The listing builds one solid part. Answer for the finished solid, in the listing's coordinates (mm). A direction names the side the tool comes from. Round coordinates to 2 decimals unless told otherwise and drop trailing zeros. Write each loop counter-clockwise with the first axis right and the second up, starting at its lowest first coordinate (ties: lowest second). Pieces come first, ordered by that corner, then holes.
(1) A cutting plane is placed at C-C, the plane y = 32. Give the vertices of the cut face in (x, z).
(2) A cutting plane is placed at B-B, the plane x = 23. Give the vertices of the cut face in (y, z).
(3) A cutting plane is placed at D-D, the plane z = 0.6. Give the vertices of the cut face in (x, y).
(4) For faces 5 (the face through (19, 8, 2)), 6 (the face through (13, 18, 3)), determine the directions among +Z, -Z, +X, -X, +Y, -Y from which every point of the face is accessible in a straight line to the end or side of a thin tool.
(5) This flat-tipped pin is pushed along its axis until it touches: pin 1 Ø4 at (x, y) = (18.5, 6) entering from +Z. Where does it stop, or does it pass through?
(6) Find the intervals of material crossed by probe 1 along X at (y, z) = (33, 1.5); probe 2 along Y at (x, z) = (18.5, 0.6); probe 3 along Y at (x, z) = (3, 0.2), in increasing order.
(7) A cutting plane is placed at A-A, the plane z = 2.55. Give the vertices of the cut face in (x, y).
(8) The mould has two halves that part along X. Classify faces 1 (the face through (25.43, 34.4, 1.48)), 2 (the face through (0.6, 34.43, 1.48)), 3 (the face through (13, 0, 1)), 4 (the face through (2.65, 30.44, 1.48)): +X half, -X half, draft (parallel to the pull), parting line (faces both ways), or undercut.
from build123d import *

# Parameters (mm, degrees)
F0_R     = 1.6
F1_DEPTH = 3
F2_DEPTH = 2


with BuildPart() as f1:
    # F0 (on Top) → F1 (new body)
    with BuildSketch(Plane.XY):
        with BuildLine():
            ThreePointArc((0, 2), (0.585786, 0.585786), (2, 0))
            Line((2, 0), (24, 0))
            ThreePointArc((24, 0), (25.414214, 0.585786), (26, 2))
            Line((26, 2), (26, 33))
            ThreePointArc((26, 33), (25.414214, 34.414214), (24, 35))
            Line((24, 35), (2, 35))
            ThreePointArc((2, 35), (0.585786, 34.414214), (0, 33))
            Line((0, 33), (0, 2))
        make_face()
        Polygon((7.5, 2.651368), (4.6, 4.325684), (4.6, 7.674316), (7.5, 9.348632), (10.4, 7.674316), (10.4, 4.325684), align=None, mode=Mode.SUBTRACT)
        Polygon((18.5, 2.651368), (15.6, 4.325684), (15.6, 7.674316), (18.5, 9.348632), (21.4, 7.674316), (21.4, 4.325684), align=None, mode=Mode.SUBTRACT)
        with Locations((3, 32)):
            Circle(F0_R, mode=Mode.SUBTRACT)
        with Locations((23, 32)):
            Circle(F0_R, mode=Mode.SUBTRACT)
    extrude(amount=F1_DEPTH)

    # F0 (on Top) → F2 (join)
    with BuildSketch(Plane.XY):
        Polygon((4.6, 7.674316), (4.6, 4.325684), (7.5, 2.651368), (10.4, 4.325684), (10.4, 7.674316), (7.5, 9.348632), align=None)
        with Locations((7.5, 6)):
            Circle(F0_R, mode=Mode.SUBTRACT)
        Polygon((15.6, 7.674316), (15.6, 4.325684), (18.5, 2.651368), (21.4, 4.325684), (21.4, 7.674316), (18.5, 9.348632), align=None)
        with Locations((18.5, 6)):
            Circle(F0_R, mode=Mode.SUBTRACT)
    extrude(amount=F2_DEPTH)


solid = f1.part
Solutions:
1. outline: (0, 0) - (1.4, 0) - (1.4, 3) - (0, 3) - close; (4.6, 0) - (21.4, 0) - (21.4, 3) - (4.6, 3) - close; (24.6, 0) - (26, 0) - (26, 3) - (24.6, 3) - close
2. outline: (0, 0) - (30.4, 0) - (30.4, 3) - (0, 3) - close; (33.6, 0) - (35, 0) - (35, 3) - (33.6, 3) - close
3. outline: (0, 2) arc R2 ccw to (2, 0) - (24, 0) arc R2 ccw to (26, 2) - (26, 33) arc R2 ccw to (24, 35) - (2, 35) arc R2 ccw to (0, 33) - close; hole circle Ø3.2 at (3, 32); hole circle Ø3.2 at (7.5, 6); hole circle Ø3.2 at (18.5, 6); hole circle Ø3.2 at (23, 32)
4. face 5: +Z
4. face 6: +Z, +X, -X, +Y, -Y
5. pin 1: stops at z = 2
6. probe 1: x = 0 to 1.75, 4.25 to 21.75, 24.25 to 26
6. probe 2: y = 0 to 4.4, 7.6 to 35
6. probe 3: y = 0 to 30.4, 33.6 to 35
7. outline: (0, 2) arc R2 ccw to (2, 0) - (24, 0) arc R2 ccw to (26, 2) - (26, 33) arc R2 ccw to (24, 35) - (2, 35) arc R2 ccw to (0, 33) - close; hole circle Ø3.2 at (3, 32); hole (4.6, 4.33) - (7.5, 2.65) - (10.4, 4.33) - (10.4, 7.67) - (7.5, 9.35) - (4.6, 7.67) - close; hole (15.6, 4.33) - (18.5, 2.65) - (21.4, 4.33) - (21.4, 7.67) - (18.5, 9.35) - (15.6, 7.67) - close; hole circle Ø3.2 at (23, 32)
8. face 1: +X half
8. face 2: -X half
8. face 3: draft
8. face 4: undercut
